Verification items for the finished model (mm, model axes). A direction names the side the tool comes from. Coordinates: 2 decimals unless noted, no trailing zeros. Loops run counter-clockwise (first coordinate to the right, second up) from the corner with the lowest first, then second, coordinate; pieces in that order, holes last.
Q1. Mould release check, pull along Y, two halves, no side actions. Record for faces 4 (the face through (-26, 2, 0)), 5 (the face through (0, 0, 0)), 6 (the face through (-20.255, 3.746, -0.056)): +Y half, -Y half, draft (parallel to the pull), parting line (faces both ways), or undercut.
Q2. Access from +Z, -Z, +X, -X, +Y, -Y to the whole of each face (thin tool, end or side, straight path). Record for faces 1 (the face through (23.465, 2.513, 0.195)), 2 (the face through (0, 4, -17.5)), 3 (the face through (-23.465, 2.513, -0.195)).
Q3. Go/stop test with a flat-tipped pin: P1, Ø1.8, axis at y = 4, z = 0, coming from the +X side. Record where the tip stops, or that it passes through.
Q4. Material ranges on probe 1 along Y at (x, z) = (-23.6, 0); probe 2 along Z at (x, y) = (-23.25, 4), recorded low to high.
Q5. Sectioned sample at A-A (x = 22). Enter the section's corners in (y, z), then the cut area to 3 significant figures.
Autodesk Inventor part; units mm, degrees
ref_plane "YZ Plane" through (0, 0, 0) normal (1, 0, 0) x (0, 1, 0)
ref_plane "XZ Plane" through (0, 0, 0) normal (0, 1, 0) x (-1, 0, 0)
ref_plane "XY Plane" through (0, 0, 0) normal (0, 0, 1) x (1, 0, 0)
sketch "Esboço1" plane through (0, 0, 0) normal (0, 1, 0) x (-1, 0, 0)
  line L0 (-26, -17.5) -> (26, -17.5)
  line L1 (26, -17.5) -> (26, 17.5)
  line L2 (26, 17.5) -> (-26, 17.5)
  line L3 (-26, 17.5) -> (-26, -17.5)
  line L4 (-26, -17.5) -> (26, 17.5) construction
  line L5 (26, -17.5) -> (-26, 17.5) construction
  point P0 (0, 0)
  dimension "d0" = 52
  dimension "d1" = 35
extrude "Extrusão1" add sketch "Esboço1" along normal blind 8
fillet "Arredondamento1" radius 1 4 edges at (26, 4, -17.5) (-26, 4, -17.5) (26, 4, 17.5) (-26, 4, 17.5)
sketch "Esboço2" plane through (-26, 0, -16.5) normal (-1, 0, 0) x (0, 0, 1)
  line L0 (0, 8) -> (33, 8)
  line L1 (0, 0) -> (33, 0)
  point P0 (16.5, 0)
  point P1 (16.5, 4)
  point P2 (16.5, 0)
  dimension "d5" = 4
hole "Furo1" at (-26, 4, 0) direction (1, 0, 0) diameter 3 depth 5 tip angle 118
sketch "Esboço3" plane through (26, 0, 16.5) normal (1, 0, 0) x (0, 0, -1)
  line L0 (0, 8) -> (33, 8)
  line L1 (0, 0) -> (33, 0)
  point P0 (16.5, 0)
  point P1 (16.5, 4)
  point P2 (16.5, 0)
  dimension "d13" = 4
hole "Furo2" at (26, 4, 0) direction (-1, 0, 0) diameter 3 depth 5 tip angle 118
properties part number "Case - Tampa" material "Plástico PC/ABS"
Geometry check:
1. face 4: draft
1. face 5: -Y half
1. face 6: undercut
2. face 1: +X
2. face 2: -Z, +X, -X, +Y, -Y
2. face 3: -X
3. P1: stops at x = 20.64
4. probe 1: y = 0 to 2.5, 5.5 to 8
4. probe 2: z = -17.5 to -1.5, 1.5 to 17.5
5. outline: (0, -17.5) - (8, -17.5) - (8, 17.5) - (0, 17.5) - close; hole circle Ø3 at (4, 0)
5. area: 273 mm2
